from build123d import *

# Parameters (mm, degrees)
SKETCH1_R           = 25.25
BOSS_EXTRUDE1_DEPTH = 5
SKETCH2_R           = 23.25
SKETCH2_R_2         = 18.25
BOSS_EXTRUDE2_DEPTH = 8
FILLET1_R           = 2.54
FILLET3_R           = 2
SKETCH3_W           = 7
SKETCH3_H           = 15
CUT_EXTRUDE1_DEPTH  = 39.001644834
SKETCH4_W           = 7
SKETCH4_H           = 3
BOSS_EXTRUDE3_DEPTH = 4
SKETCH5_W           = 7
SKETCH5_H           = 21
BOSS_EXTRUDE4_DEPTH = 2
FILLET4_R           = 2
FILLET5_R           = 1
FILLET6_START       = -12.5
FILLET6_DEPTH       = 5
FILLET6_START_2     = 7.5
FILLET6_2_DEPTH     = 5
FILLET6_START_3     = -6
FILLET6_3_DEPTH     = 12


with BuildPart() as part:
    # Sketch1 → Boss-Extrude1 (new body)
    with BuildSketch(Plane(origin=(0, 0, 0), x_dir=(1, 0, 0), z_dir=(0, 1, 0))):
        with Locations(Location((0, 0, 0), (0, 0, 270))):
            Circle(SKETCH1_R)
    extrude(amount=BOSS_EXTRUDE1_DEPTH)

    # Sketch2 → Boss-Extrude2 (add)
    with BuildSketch(Plane(origin=(0, 5, 0), x_dir=(1, 0, 0), z_dir=(0, 1, 0))):
        with Locations(Location((0, 0, 0), (0, 0, 270))):
            Circle(SKETCH2_R)
        with Locations(Location((0, 0, 0), (0, 0, 270))):
            Circle(SKETCH2_R_2, mode=Mode.SUBTRACT)
    extrude(amount=BOSS_EXTRUDE2_DEPTH)

    # Fillet1
    fillet1_edges = [part.edges().sort_by_distance(p)[0] for p in [
        (0, 0, -25.25),
        (0, 5, -18.25),
    ]]
    fillet(fillet1_edges, radius=FILLET1_R)

    # Fillet3
    fillet3_edges = [part.edges().sort_by_distance(p)[0] for p in [
        (0, 13, -23.25),
    ]]
    fillet(fillet3_edges, radius=FILLET3_R)

    # Sketch3 → Cut-Extrude1 (cut, through all)
    with BuildSketch(Plane(origin=(0, 0, 0), x_dir=(-1, 0, 0), z_dir=(0, -1, 0))):
        Rectangle(SKETCH3_W, SKETCH3_H)
    extrude(amount=-CUT_EXTRUDE1_DEPTH, mode=Mode.SUBTRACT)

    # Sketch4 → Boss-Extrude3 (add)
    with BuildSketch(Plane(origin=(0, 0, 0), x_dir=(-1, 0, 0), z_dir=(0, -1, 0))):
        with Locations((0, 9)):
            Rectangle(SKETCH4_W, SKETCH4_H)
        with Locations((0, -9)):
            Rectangle(SKETCH4_W, SKETCH4_H)
    extrude(amount=BOSS_EXTRUDE3_DEPTH)

    # Sketch5 → Boss-Extrude4 (add)
    with BuildSketch(Plane(origin=(0, -4, 0), x_dir=(-1, 0, 0), z_dir=(0, -1, 0))):
        Rectangle(SKETCH5_W, SKETCH5_H)
    extrude(amount=BOSS_EXTRUDE4_DEPTH)

    # Fillet4
    fillet4_edges = [part.edges().sort_by_distance(p)[0] for p in [
        (0, 0, -10.5),
        (0, 0, 10.5),
    ]]
    fillet(fillet4_edges, radius=FILLET4_R)

    # Fillet5
    fillet5_edges = [part.edges().sort_by_distance(p)[0] for p in [
        (0, -4, -7.5),
        (0, -4, 7.5),
    ]]
    fillet(fillet5_edges, radius=FILLET5_R)

    # Fillet6: read off the stored shape, not the designer's step
    # Fillet6 outline → Fillet6 (add)
    with BuildSketch(Plane.XY.offset(FILLET6_START)):
        with BuildLine():
            Line((5.5, 0), (3.5, 0))
            Line((3.5, 0), (3.5, -2))
            ThreePointArc((3.5, -2), (4.085786438, -0.585786438), (5.5, 0))
        make_face()
        with BuildLine():
            ThreePointArc((-5.5, 0), (-4.085786438, -0.585786438), (-3.5, -2))
            Line((-3.5, -2), (-3.5, 0))
            Line((-3.5, 0), (-5.5, 0))
        make_face()
    extrude(amount=FILLET6_DEPTH)

    # Fillet6 2 outline → Fillet6 2 (add)
    with BuildSketch(Plane.XY.offset(FILLET6_START_2)):
        with BuildLine():
            Line((5.5, 0), (3.5, 0))
            Line((3.5, 0), (3.5, -2))
            ThreePointArc((3.5, -2), (4.085786438, -0.585786438), (5.5, 0))
        make_face()
        with BuildLine():
            ThreePointArc((-5.5, 0), (-4.085786438, -0.585786438), (-3.5, -2))
            Line((-3.5, -2), (-3.5, 0))
            Line((-3.5, 0), (-5.5, 0))
        make_face()
    extrude(amount=FILLET6_2_DEPTH)

    # Fillet6 3 outline → Fillet6 3 (cut)
    with BuildSketch(Plane.YZ.offset(FILLET6_START_3)):
        with BuildLine():
            Line((-2, -10.5), (-2, -12.5))
            Line((-2, -12.5), (0, -12.5))
            ThreePointArc((0, -12.5), (-0.585786438, -11.085786438), (-2, -10.5))
        make_face()
        with BuildLine():
            Line((-2, 12.5), (-2, 10.5))
            ThreePointArc((-2, 10.5), (-0.585786438, 11.085786438), (0, 12.5))
            Line((0, 12.5), (-2, 12.5))
        make_face()
    extrude(amount=FILLET6_3_DEPTH, mode=Mode.SUBTRACT)


solid = part.part
The model under review builds one solid part; all positions refer to its coordinate system, in mm. A direction names the side the tool comes from. Coordinates: 2 decimals unless noted, no trailing zeros. Loops run counter-clockwise (first coordinate to the right, second up) from the corner with the lowest first, then second, coordinate; pieces in that order, holes last. Notation, with made-up numbers: M 36.5,43 L 49.5,43 A16 ccw 49.5,67 Z; hole C 23,-24.75 d10. An arc over 180 degrees is marked long. Put each result on its own line as item: value. Start each with the question number.
Q1. For faces 4 (the cylindrical face through (23.05, 7.96, -3.03)), 5 (the flat face through (3.5, -4.4, 0.1)), 6 (the flat face through (0, -4, -10.5)), 7 (the flat face through (-3.5, -4.4, 0.1)), list the 3-axis set-ups (+Z, -Z, +X, -X, +Y, -Y) from which the entire face can be reached by the end or side of a thin tool; tool diameter is ignored.
Q2. Add section C-C (y = 4.25). Write out the cut boundary in (x, z).
Q3. The part is to be moulded in two halves that separate along X. For faces 1 (the cylindrical face through (-15.36, 3.75, -20.04)), 2 (the flat face through (3.5, 2, 0)), 3 (the flat face through (0, -4, 10.5)), say which applies: +X half, -X half, draft (parallel to the pull), parting line (faces both ways), or undercut.
Q4. Wall thickness on line 1 (X direction, y = 11.1, z = 0); line 2 (Y direction, x = -8, z = 13.5); line 3 (Y direction, x = -0.5, z = -21): over which ranges is each line inside the solid? List them lowest first.
Q5. Add section A-A (z = 0). Write out the cut boundary in (x, y).
Q6. Clearance check with flat-ended pins moving along their axes: pin 1 (2 mm diameter, centred on x = -0.5, z = -0.5, fed in from +Y); pin 2 (4 mm diameter, centred on y = 6, z = -16, fed in from -X); pin 3 (3 mm diameter, centred on y = -4, z = -4, fed in from -X). State where each tip first meets the part, or that it passes through.
Answers:
1. face 4: +Y
1. face 5: +Z, -Z, +X, -Y
1. face 6: -Z, +X, -X, -Y
1. face 7: +Z, -Z, -X, -Y
2. outline: C 0,0 d50.5; hole M -3.5,-7.5 L 3.5,-7.5 L 3.5,7.5 L -3.5,7.5 Z
3. face 1: parting line
3. face 2: undercut
3. face 3: draft
4. line 1: x = -23.25 to -18.25, 18.25 to 23.25
4. line 2: y = 0 to 5
4. line 3: y = 0 to 13
5. outline: M -25.25,2.54 A2.54 ccw -22.71,0 L -3.5,0 L -3.5,5 L -15.71,5 A2.54 cw -18.25,7.54 L -18.25,13 L -21.25,13 A2 ccw -23.25,11 L -23.25,5 L -25.25,5 Z; M -3.5,-6 L 3.5,-6 L 3.5,-4 L -3.5,-4 Z; M 3.5,0 L 22.71,0 A2.54 ccw 25.25,2.54 L 25.25,5 L 23.25,5 L 23.25,11 A2 ccw 21.25,13 L 18.25,13 L 18.25,7.54 A2.54 cw 15.71,5 L 3.5,5 Z
6. pin 1: stops at y = -4
6. pin 2: stops at x = -20.83
6. pin 3: stops at x = -3.5
